Design review of the part built by this model. Coordinates are the model's own, in mm. Face numbers are marked on the shaded views. Give positions to 0.01 mm unless a question says otherwise; leave off trailing zeros. Order: outer loops, then holes, each group sorted by start corner. A loop starts at its lowest first (then second) coordinate and runs counter-clockwise, first axis right, second up. Notation, with made-up numbers: M 20,32 L 28,32 A23 ccw 28,65 Z; hole C 72.5,65 d2. An arc over 180 degrees is marked long. Answer as a JSON object with one key per item and string values.
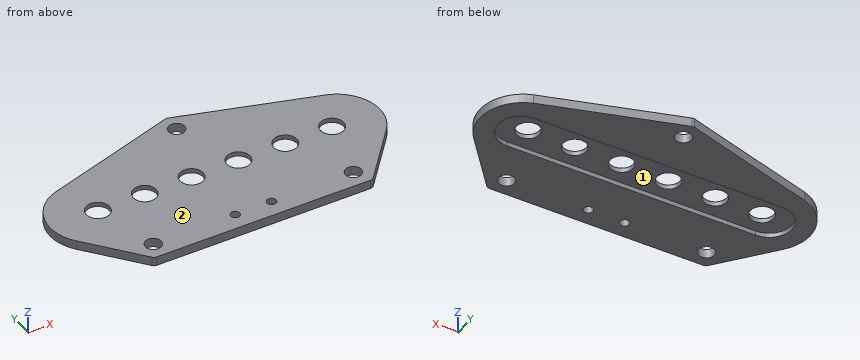
Autodesk Fusion 360 part; units mm, degrees
sketch "スケッチ1" plane through (0, 0, 0) normal (0, 0, 1) x (1, 0, 0)
  line L0 (0, 0) -> (72.6, 0)
  line L1 (72.6, 0) -> (72.6, -36.25)
  line L2 (72.6, -36.25) -> (0, -36.25)
  line L3 (0, -36.25) -> (0, 0)
  line L4 (36.3, 0) -> (36.3, -36.25)
  line L5 (0, -18.125) -> (72.6, -18.125)
  line L6 (72.6, -8.625) -> (72.6, -26.625)
  line L7 (58.3, -36.25) -> (14.3, -36.25)
  line L8 (0, -9.125) -> (0, -27.125)
  line L9 (0, -18.125) -> (9.5, -18.125)
  line L10 (0, -9.125) -> (6.4586, -9.125)
  line L11 (0, -27.125) -> (4.6488, -27.125)
  line L12 (6.4586, -9.125) -> (36.3, 0)
  line L13 (14.3, -36.25) -> (12.3, -36.25)
  line L14 (12.3, -36.25) -> (2.2204, -24.2289)
  line L15 (36.3, -18.125) -> (36.3, -32.425)
  line L16 (36.3, -18.125) -> (36.3, -3.825)
  line L17 (66.1414, -9.125) -> (36.3, 0)
  line L18 (60.3, -36.25) -> (70.3796, -24.2289)
  line L19 (58.3, -36.25) -> (60.3, -36.25)
  line L20 (6.4586, -27.125) -> (66.1414, -27.125)
  line L21 (6.4586, -9.125) -> (66.1414, -9.125)
  arc A0 (6.9878, -8.9632) -> (6.4586, -27.125) centre (9.5, -18.125) ccw
  arc A1 (66.1414, -27.125) -> (65.6122, -8.9632) centre (63.1, -18.125) ccw
  circle A2 centre (14.3, -32.425) radius 1.75
  circle A3 centre (36.3, -3.825) radius 1.75
  circle A4 centre (58.3, -32.425) radius 1.75
  circle A5 centre (32.3, -32.425) radius 1
  circle A6 centre (40.3, -32.425) radius 1
  line L22 (36.3, -9.125) -> (36.3, -13.125)
  line L23 (0, -18.125) -> (4, -18.125)
  line L24 (36.3, -13.125) -> (5.4223, -13.125)
  line L25 (36.3, -27.125) -> (36.3, -23.125)
  line L26 (36.3, -23.125) -> (5.4223, -23.125)
  arc A7 (5.4223, -13.125) -> (5.4223, -23.125) centre (13.5, -18.125) ccw
  circle A8 centre (10.55, -18.125) radius 2.55
  circle A9 centre (20.85, -18.125) radius 2.55
  circle A10 centre (31.15, -18.125) radius 2.55
  line L27 (36.3, -13.125) -> (67.1777, -13.125)
  arc A11 (67.1777, -23.125) -> (67.1777, -13.125) centre (59.1, -18.125) ccw
  line L28 (36.3, -23.125) -> (67.1777, -23.125)
  circle A12 centre (41.45, -18.125) radius 2.55
  circle A13 centre (51.75, -18.125) radius 2.55
  circle A14 centre (62.05, -18.125) radius 2.55
  point P0 (36.3, -18.125)
  point P1 (36.3, -3.825)
  point P2 (14.3, -32.425)
  point P3 (58.3, -32.425)
  point P4 (40.3, -32.425)
  point P5 (40.3, -32.425)
  point P6 (32.3, -32.425)
  point P7 (31.15, -18.125)
  point P8 (20.85, -18.125)
  point P9 (10.55, -18.125)
  point P10 (41.45, -18.125)
  point P11 (51.75, -18.125)
  point P12 (62.05, -18.125)
  dimension "d5" = 72.6
  dimension "d6" = 36.25
  dimension "d10" = 44
  dimension "d11" = 9
  dimension "d12" = 18
  dimension "d13" = 9.5
  dimension "d14" = 2
  dimension "d15" = 14.3
  dimension "d16" = 22
  dimension "d17" = 14.3
  dimension "d18" = 3.5
  dimension "d19" = 3.5
  dimension "d20" = 3.5
  dimension "d21" = 4
  dimension "d24" = 2
  dimension "d25" = 2
  dimension "d30" = 4
  dimension "d31" = 4
  dimension "d32" = 9.5
  dimension "d33" = 4
  dimension "d34" = 5.15
  dimension "d35" = 10.3
  dimension "d36" = 10.3
  dimension "d37" = 5.1
  dimension "d38" = 5.1
  dimension "d39" = 5.1
  dimension "d46" = 5.1
  dimension "d47" = 5.1
  dimension "d48" = 5.1
extrude "押し出し1" add sketch "スケッチ1" along normal blind 2 contours L4 L16 L17 L21 A3 | L4 L12 L16 L21 A3 | L4 L5 L9 L16 L21 A0 L22 L23 L24 A7 | L4 L5 L9 L15 L20 A0 L23 L25 L26 A7 | L4 L5 L16 L21 A1 L22 L27 A11 | L4 L5 L9 L16 L24 A7 A8 A9 A10 | L4 L5 L9 L15 L26 A7 A8 A9 A10 | L2 L4 L7 L13 L14 L15 L20 A0 | L4 L5 L15 L20 A1 L25 A11 L28 | L5 L9 A8 | L5 L9 A8 | L4 L5 L16 L27 A11 A12 A13 A14 | L4 L5 L15 A11 L28 A12 A13 A14 | L2 L4 L7 L15 L18 L19 L20 A1 | L5 A14 | L5 A14 | L5 A9 | L5 A9 | L5 A10 | L5 A10 | L5 A12 | L5 A12 | L5 A13 | L5 A13
fillet "フィレット1" radius 1 3 edges at (12.3, -36.25, 1) (60.3, -36.25, 1) (36.3, 0, 1)
sketch "スケッチ2" plane through (0, 0, 2) normal (0, 0, 1) x (-1, 0, 0)
  arc A0 (-36.5924, 0.0894) -> (-36.0076, 0.0894) centre (-36.3, 1.0457) ccw
  line L0 (-36.0076, 0.0894) -> (-6.4586, 9.125)
  arc A1 (-6.4586, 9.125) -> (-2.2204, 24.2289) centre (-9.5, 18.125) ccw
  line L1 (-2.2204, 24.2289) -> (-12.0003, 35.8925)
  arc A2 (-12.0003, 35.8925) -> (-12.7665, 36.25) centre (-12.7665, 35.25) ccw
  line L2 (-12.7665, 36.25) -> (-59.8335, 36.25)
  arc A3 (-59.8335, 36.25) -> (-60.5997, 35.8925) centre (-59.8335, 35.25) ccw
  line L3 (-60.5997, 35.8925) -> (-70.3796, 24.2289)
  arc A4 (-70.3796, 24.2289) -> (-66.1414, 9.125) centre (-63.1, 18.125) ccw
  line L4 (-66.1414, 9.125) -> (-36.5924, 0.0894)
  circle A5 centre (-36.3, 3.825) radius 1.75
  circle A6 centre (-32.3, 32.425) radius 1
  circle A7 centre (-40.3, 32.425) radius 1
  circle A8 centre (-14.3, 32.425) radius 1.75
  circle A9 centre (-58.3, 32.425) radius 1.75
extrude "押し出し2" cut sketch "スケッチ1" along normal blind 2 contours L5 L9 A8 | L5 L9 A8 | L5 A14 | L5 A14 | L5 A9 | L5 A9 | L5 A10 | L5 A10 | L5 A12 | L5 A12 | L5 A13 | L5 A13
extrude "押し出し3" cut sketch "スケッチ1" along normal blind 1 contours L4 L5 L9 L16 L24 A7 A8 A9 A10 | L4 L5 L9 L15 L26 A7 A8 A9 A10 | L5 L9 A8 | L5 L9 A8 | L4 L5 L16 L27 A11 A12 A13 A14 | L4 L5 L15 A11 L28 A12 A13 A14 | L5 A14 | L5 A14 | L5 A9 | L5 A9 | L5 A10 | L5 A10 | L5 A12 | L5 A12 | L5 A13 | L5 A13
fillet "フィレット2" radius 5 4 edges at (5.4223, -23.125, 0.5) (5.4223, -13.125, 0.5) (67.1777, -23.125, 0.5) (67.1777, -13.125, 0.5)
(1) To check wall thickness, follow L1, parallel to Y at x = 32.5, z = 1.95; L2, parallel to Y at x = 40.3, z = 0.85 (3 decimals); L3, parallel to Y at x = 22, z = 0.95 (3 decimals). State the ranges of each line that lie inside material, in increasing order. Write a range as from..to.
Checked values:
{"L1": "y = -36.25..-33.4, -31.45..-20.29, -15.96..-1.16", "L2": "y = -36.25..-33.425, -31.425..-23.125, -13.125..-1.223", "L3": "y = -36.25..-23.125, -13.125..-4.373"}
(2) We need section C-C (x = 51). Write out the cut boundary in (y, z) (3 decimals).
Checked values:
{"outline": "M -36.25,0 L -23.125,0 L -23.125,1 L -20.562,1 L -20.562,2 L -36.25,2 Z; M -15.688,1 L -13.125,1 L -13.125,0 L -4.495,0 L -4.495,2 L -15.688,2 Z"}
(3) We need section A-A (x = 40.3). Write out the cut boundary in (y, z) (3 decimals), plus the area to 3 significant figures.
Checked values:
{"outline": "M -36.25,0 L -33.425,0 L -33.425,2 L -36.25,2 Z; M -31.425,0 L -23.125,0 L -23.125,1 L -20.401,1 L -20.401,2 L -31.425,2 Z; M -15.849,1 L -13.125,1 L -13.125,0 L -1.223,0 L -1.223,2 L -15.849,2 Z", "area": "51.5 mm^2"}
(4) Insertion check: pin 1 (3 mm diameter, centred on x = 23.5, y = -18, fed in from -Z); pin 2 (0.8 mm diameter, centred on x = 39.5, z = 0.5, fed in from +Y). Each pin has a flat end and moves straight along its axis. Give the tip position at first contact, or say it passes through.
Checked values:
{"pin 1": "stops at z = 1", "pin 2": "stops at y = -0.86"}
(5) We need section B-B (y = -19.5). Count the separate pieces of the cut face and the enclosed holes in it, plus the area to 3 significant figures.
Checked values:
{"separate pieces": "7", "enclosed holes": "0", "area": "54.8 mm^2"}
(6) Draft analysis for pull direction Y (two halves, no side actions). For the marked faces 1 and 2, state which applies: +Y half, -Y half, draft (parallel to the pull), parting line (faces both ways), or undercut.
Checked values:
{"face 1": "undercut", "face 2": "draft"}
(7) We need section D-D (y = -14.5). Write out the cut boundary in (x, z).
Checked values:
{"outline": "M 0.72,0 L 5.56,0 L 5.56,1 L 67.04,1 L 67.04,0 L 71.88,0 L 71.88,2 L 0.72,2 Z"}
